Study the drawing (mm; zero at the part's minimum x, y, z) and answer. Coordinates: 2 decimals unless noted, no trailing zeros. Order: outer loops, then holes, each group sorted by start corner. A loop starts at its lowest first (then second) coordinate and runs counter-clockwise, first axis right, second up.
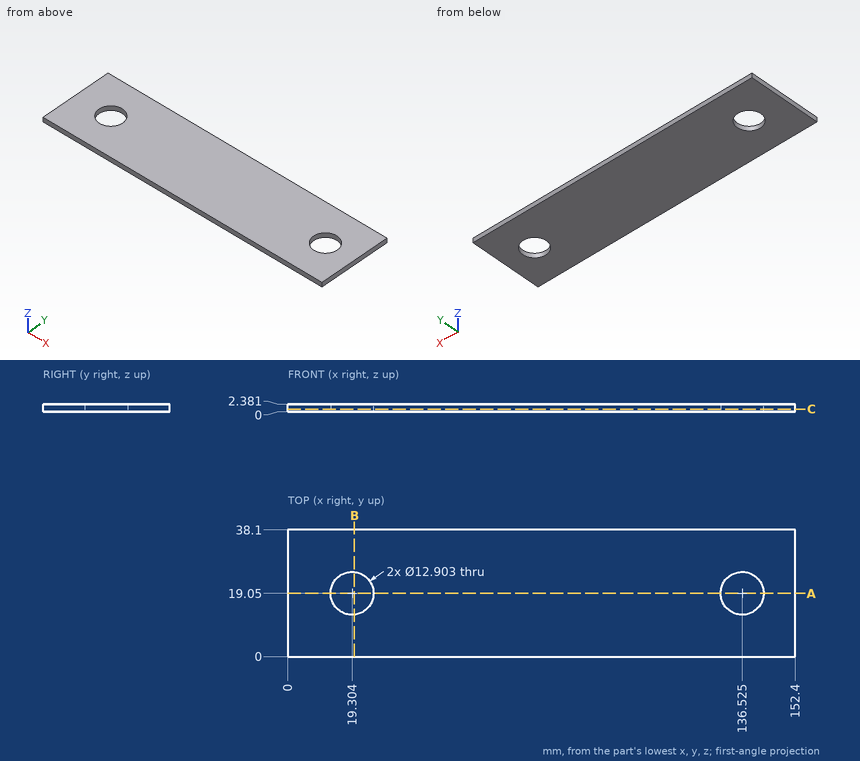
1) A cutting plane is placed at C-C, the plane z = 0.85. State how many separate pieces and enclosed holes the cut face has, and give its area (4 significant figures).
A:
separate pieces: 1
enclosed holes: 2
area: 5,545 mm2
2) A flat-ended cylindrical pin translates along its axis: pin 1 Ø10 at (x, y) = (95, 27.5) entering from -Z. Find the tip coordinate at first contact, or state that the pin passes through.
A:
pin 1: stops at z = 0
3) A cutting plane is placed at B-B, the plane x = 20. Determine the outline of the cut face in (y, z).
A:
outline: (0, 0) - (12.64, 0) - (12.64, 2.38) - (0, 2.38) - close; (25.46, 0) - (38.1, 0) - (38.1, 2.38) - (25.46, 2.38) - close
4) A cutting plane is placed at A-A, the plane y = 19.05. Determine the outline of the cut face in (x, z).
A:
outline: (0, 0) - (12.85, 0) - (12.85, 2.38) - (0, 2.38) - close; (25.76, 0) - (130.07, 0) - (130.07, 2.38) - (25.76, 2.38) - close; (142.98, 0) - (152.4, 0) - (152.4, 2.38) - (142.98, 2.38) - close
5) Straight lines are drawn through the part: line 1 (X direction, y = 19.05, z = 1.5); line 2 (X direction, y = 21, z = 0.55) (1 decimal); line 3 (Y direction, x = 19.5, z = 0.45). For each, find the intervals that lie inside material, in ascending order.
A:
line 1: x = 0 to 12.85, 25.76 to 130.07, 142.98 to 152.4
line 2: x = 0 to 13.2, 25.5 to 130.4, 142.7 to 152.4
line 3: y = 0 to 12.6, 25.5 to 38.1
